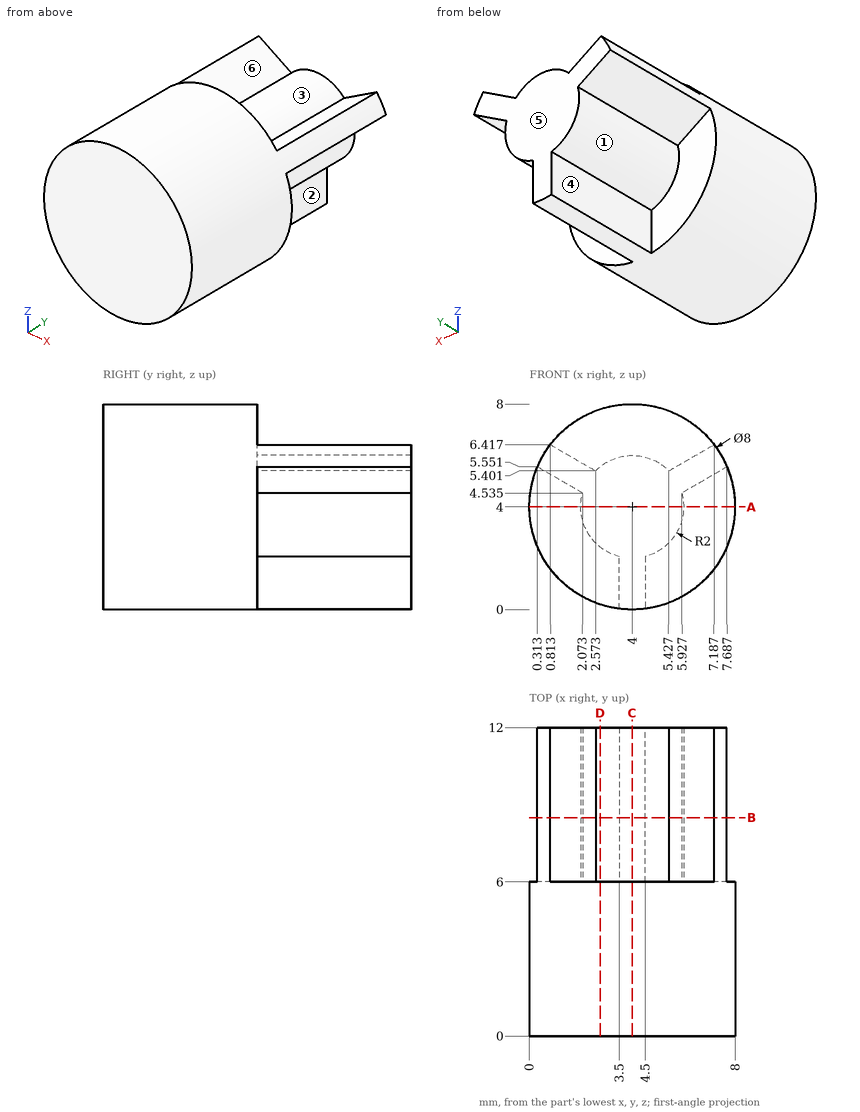
Print and shaded views of the part. All mm, measured from the part's lowest x, y and z. A direction names the side the tool comes from. Coordinates: 2 decimals unless noted, no trailing zeros. Loops run counter-clockwise (first coordinate to the right, second up) from the corner with the lowest first, then second, coordinate; pieces in that order, holes last. Notation, with made-up numbers: (59.25, -36) - (78.25, -36) arc R20 cw to (78.25, -26) - close; hole circle Ø9 at (-38.5, -6). An arc over 180 degrees is marked (long way). Write item = value, one per line. Start each with the question number.
Item 1: Wall check: L1, parallel to Y at x = 3, z = 0.75; L2, parallel to X at y = 10, z = 4; L3, parallel to X at y = 9.75, z = 2. Give the ranges that are in metal, low to high. Write a range as from..to.
Item 2: Mould opens along X. For the marked faces 1, 2 and 3 say: released by +X, released by -X, zero draft, split by the parting line, or undercut.
Item 3: Cut at B-B, the plane y = 8.5. Give the cut face in (x, z) (1 decimal).
Item 4: 3-axis set-ups, long thin cutter, end or side, ignore diameter. For the marked faces 4, 5 and 6: which of +Z, -Z, +X, -X, +Y, -Y reach the whole face in a straight line?
Item 5: Cut at C-C, the plane x = 4. Give the cut face in (y, z), and give its area (3 significant figures).
Item 6: Cut at A-A, the plane z = 4. Give the cut face in (x, y).
Item 7: Flat gauge pins, fed straight in: pin 1 Ø0.6 at (y, z) = (9, 1.5) entering from +X; pin 2 Ø1 at (y, z) = (10, 0.5) entering from -X; pin 3 Ø1.8 at (x, z) = (1, 3.5) entering from +Y. Where does each tip first touch, or does it go through?
Item 8: Cut at D-D, the plane x = 2.75. Give the cut face in (y, z).
The answers:
q1.L1 = 0..6
q1.L2 = 2..6
q1.L3 = 3.5..4.5
q2.face_1 = released by -X
q2.face_2 = released by +X
q2.face_3 = undercut
q3.outline = (0.3, 5.6) - (2.1, 4.5) arc R2 ccw to (3.5, 2.1) - (3.5, 0) arc R4 ccw to (4.5, 0) - (4.5, 2.1) arc R2 ccw to (5.9, 4.5) - (7.7, 5.6) arc R4 ccw to (7.2, 6.4) - (5.4, 5.4) arc R2 ccw to (2.6, 5.4) - (0.8, 6.4) arc R4 ccw to start
q4.face_4 = -Z, -X, +Y
q4.face_5 = +Z, -Z, +X, -X, +Y
q4.face_6 = +Z, +Y
q5.outline = (0, 0) - (12, 0) - (12, 6) - (6, 6) - (6, 8) - (0, 8) - close
q5.area = 84.0 mm2
q6.outline = (0, 0) - (8, 0) - (8, 6) - (6, 6) - (6, 12) - (2, 12) - (2, 6) - (0, 6) - close
q7.pin_1 = 4.5
q7.pin_2 = 3.5
q7.pin_3 = 6
q8.outline = (0, 0.2) - (6, 0.2) - (6, 2.44) - (12, 2.44) - (12, 5.56) - (6, 5.56) - (6, 7.8) - (0, 7.8) - close
